Answer from the drawing. Dimensions are ordinates in mm from the lowest x, y and z of the part. Give positions to 0.01 mm unless a question says otherwise; leave off trailing zeros. Order: outer loops, then holes, each group sorted by start corner. A loop starts at its lowest first (then second) coordinate and runs counter-clockwise, first axis right, second up. Notation, with made-up numbers: (11.5, -4) - (66.5, -4) arc R8 ccw to (66.5, 11) - close; hole circle Ø10 at (11, 71.25). An arc over 180 degrees is marked (long way). Write each question's results on one line, items separated by ' | '.
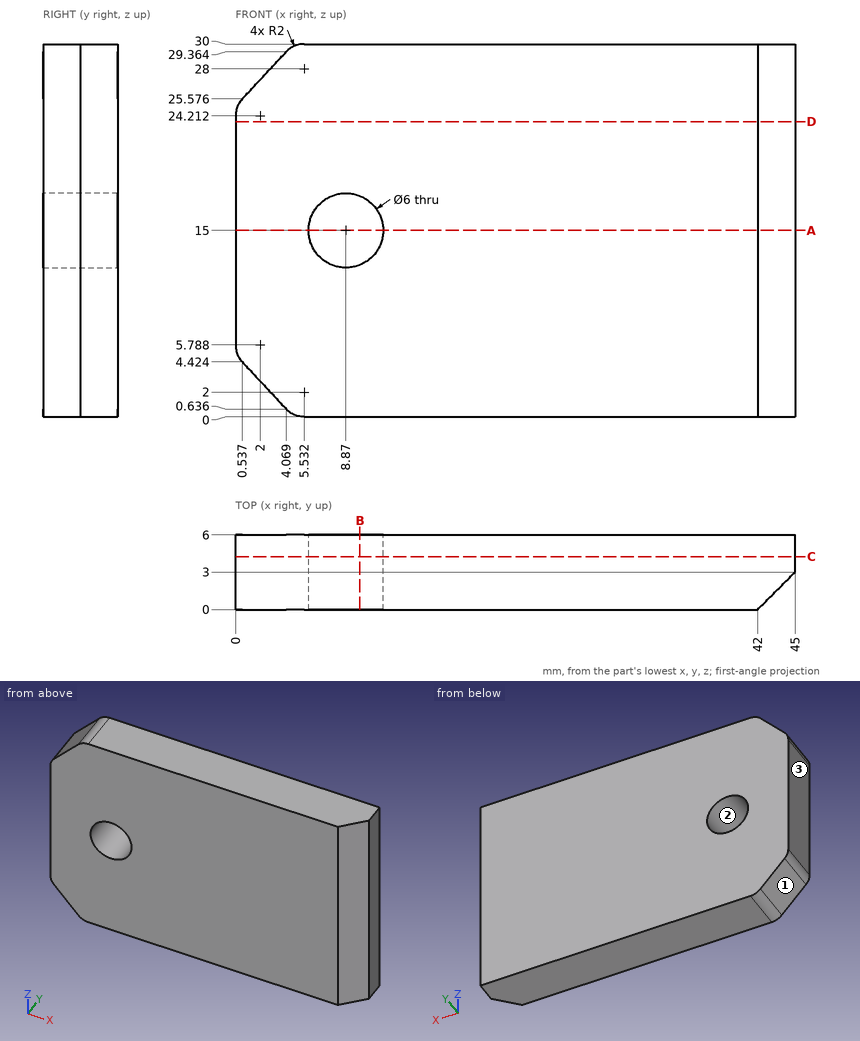
(1) Section C-C (y = 4.25) is taken. Give the vertices of the cut face in (x, z).
Conclusion:
outline: (0, 5.79) arc R2 ccw to (0.54, 4.42) - (4.07, 0.64) arc R2 ccw to (5.53, 0) - (45, 0) - (45, 30) - (5.53, 30) arc R2 ccw to (4.07, 29.36) - (0.54, 25.58) arc R2 ccw to (0, 24.21) - close; hole circle Ø6 at (8.87, 15)
(2) Section D-D (z = 23.75) is taken. Give the vertices of the cut face in (x, y).
Conclusion:
outline: (0, 0) - (42, 0) - (45, 3) - (45, 6) - (0, 6) - close
(3) Consider probe 1 along X at (y, z) = (3.2, 15); probe 2 along Z at (x, y) = (9, 3); probe 3 along X at (y, z) = (2.5, 17.5) (1 decimal). Determine where each line is inside the solid, lowest interval first. Write a range as [from, to].
Conclusion:
probe 1: [0, 5.87], [11.87, 45] | probe 2: [0, 12], [18, 30] | probe 3: [0, 7.2], [10.5, 44.5]
(4) Section B-B (x = 10) is taken. Give the vertices of the cut face in (y, z).
Conclusion:
outline: (0, 0) - (6, 0) - (6, 12.22) - (0, 12.22) - close; (0, 17.78) - (6, 17.78) - (6, 30) - (0, 30) - close
(5) The mould has two halves that part along Z. Classify the marked faces 1, 2 and 3: pulls with the +Z half, pulls with the -Z half, needs draft (parallel to the pull), parting line crosses it, or undercut.
Conclusion:
face 1: pulls with the -Z half | face 2: undercut | face 3: needs draft
(6) Section A-A (z = 15) is taken. Give the vertices of the cut face in (x, y).
Conclusion:
outline: (0, 0) - (5.87, 0) - (5.87, 6) - (0, 6) - close; (11.87, 0) - (42, 0) - (45, 3) - (45, 6) - (11.87, 6) - close
